Verification items for the finished model (mm, model axes). Coordinates: 2 decimals unless noted, no trailing zeros. Order: outer loops, then holes, each group sorted by start corner. A loop starts at its lowest first (then second) coordinate and runs counter-clockwise, first axis right, second up. Notation, with made-up numbers: M 4.5,-37 L 61.5,-37 A31 ccw 61.5,-13 Z; hole C 61.5,-13 d11. An arc over 180 degrees is marked long. Write item = value, one per line.
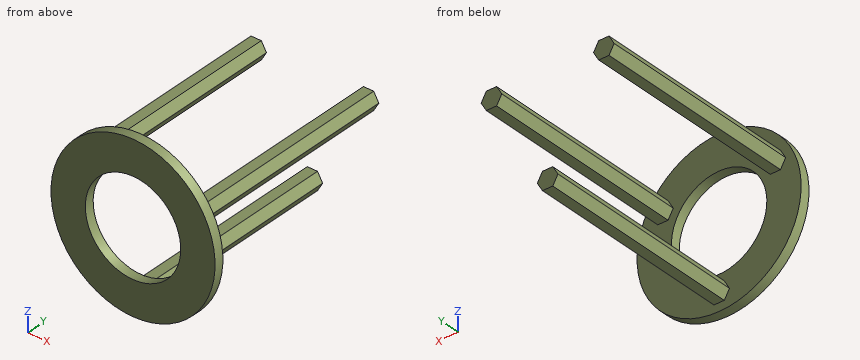
```python
from build123d import *

# Parameters (mm, degrees)
SKETCH_1_R      = 27.5
SKETCH_1_R_2    = 16
EXTRUDE_1_DEPTH = 3.2
EXTRUDE_2_DEPTH = 70


with BuildPart() as part:
    # Эскиз1 → Бобышка-Вытянуть1 (new body)
    with BuildSketch(Plane(origin=(0, 0, 0), x_dir=(1, 0, 0), z_dir=(0, 1, 0))):
        with Locations(Location((0, 0, 0), (0, 0, 270))):
            Circle(SKETCH_1_R)
        with Locations(Location((0, 0, 0), (0, 0, 270))):
            Circle(SKETCH_1_R_2, mode=Mode.SUBTRACT)
    extrude(amount=EXTRUDE_1_DEPTH)

    # Эскиз2 → Бобышка-Вытянуть2 (add)
    with BuildSketch(Plane(origin=(0, 3.2, 0), x_dir=(1, 0, 0), z_dir=(0, 1, 0))):
        Polygon((17.104001725, -13.875), (20.56810334, -13.875), (22.300154147, -10.875), (20.56810334, -7.875), (17.104001725, -7.875), (15.371950917, -10.875), align=None)
        Polygon((3.464101615, 21.75), (1.732050808, 24.75), (-1.732050808, 24.75), (-3.464101615, 21.75), (-1.732050808, 18.75), (1.732050808, 18.75), align=None)
        Polygon((-20.56810334, -7.875), (-22.300154147, -10.875), (-20.56810334, -13.875), (-17.104001725, -13.875), (-15.371950917, -10.875), (-17.104001725, -7.875), align=None)
    extrude(amount=EXTRUDE_2_DEPTH)


solid = part.part
```
Item 1: Sectioned sample at B-B, the plane z = 0. Enter the section's corners in (x, y).
Report:
outline = M -27.5,0 L -16,0 L -16,3.2 L -27.5,3.2 Z; M 16,0 L 27.5,0 L 27.5,3.2 L 16,3.2 Z
Item 2: Sectioned sample at A-A, the plane x = 0. Enter the section's corners in (y, z), then the cut area to 3 significant figures.
Report:
outline = M 0,-27.5 L 3.2,-27.5 L 3.2,-24.75 L 73.2,-24.75 L 73.2,-18.75 L 3.2,-18.75 L 3.2,-16 L 0,-16 Z; M 0,16 L 3.2,16 L 3.2,27.5 L 0,27.5 Z
area = 494 mm^2
Item 3: Scan lines: L1, parallel to X at y = 1, z = 0; L2, parallel to Z at x = -20, y = 54 (3 decimals); L3, parallel to Y at x = 23.5, z = -4. Record each from-to range of solid material in increasing order. Write a range as from..to.
Report:
L1 = -27.5..-16, 16..27.5
L2 = 7.875..13.875
L3 = 0..3.2
Item 4: Gauge pin test, flat ends, axial feed: pin 1 (10 mm diameter, centred on y = 13, z = -3.5, fed in from -X); pin 2 (12 mm diameter, centred on x = 11.5, y = 39.5, fed in from -Z) (3 decimals); pin 3 (1 mm diameter, centred on x = -0.5, y = 25.5, fed in from -Z); pin 4 (1.7 mm diameter, centred on x = 18.5, y = 28.5, fed in from +Z) (3 decimals). Record the tip position at first contact, or that the pin passes through.
Report:
pin_1 = through
pin_2 = 7.875
pin_3 = -24.75
pin_4 = 13.875
Item 5: Sectioned sample at D-D, the plane x = 13. Enter the section's corners in (y, z), then the cut area to 3 significant figures.
Report:
outline = M 0,-24.23 L 3.2,-24.23 L 3.2,-9.33 L 0,-9.33 Z; M 0,9.33 L 3.2,9.33 L 3.2,24.23 L 0,24.23 Z
area = 95.4 mm^2
Item 6: Sectioned sample at C-C, the plane y = 41. Enter the section's corners in (x, z) (3 decimals).
Report:
outline = M -22.3,10.875 L -20.568,7.875 L -17.104,7.875 L -15.372,10.875 L -17.104,13.875 L -20.568,13.875 Z; M -3.464,-21.75 L -1.732,-24.75 L 1.732,-24.75 L 3.464,-21.75 L 1.732,-18.75 L -1.732,-18.75 Z; M 15.372,10.875 L 17.104,7.875 L 20.568,7.875 L 22.3,10.875 L 20.568,13.875 L 17.104,13.875 Z
